The model under review builds one solid part; all positions refer to its coordinate system, in mm. A direction names the side the tool comes from. Round coordinates to 2 decimals unless told otherwise and drop trailing zeros. Order: outer loops, then holes, each group sorted by start corner. A loop starts at its lowest first (then second) coordinate and runs counter-clockwise, first axis right, second up.
Autodesk Inventor part; units mm, degrees
ref_plane "YZ Plane" through (0, 0, 0) normal (1, 0, 0) x (0, 1, 0)
ref_plane "XZ Plane" through (0, 0, 0) normal (0, 1, 0) x (-1, 0, 0)
ref_plane "XY Plane" through (0, 0, 0) normal (0, 0, 1) x (1, 0, 0)
sketch "Sketch1" plane through (0, 0, 0) normal (0, 0, 1) x (1, 0, 0)
  circle A0 centre (0, 0) radius 100
  dimension "Dia" = 200
extrude "Extrusion1" add sketch "Sketch1" along normal blind 25
sketch "Sketch2" plane through (0, 0, 25) normal (0, 0, 1) x (1, 0, 0)
  line L0 (-100, 12.5) -> (100, 12.5)
  line L1 (100, 12.5) -> (100, -12.5)
  line L2 (100, -12.5) -> (-100, -12.5)
  line L3 (-100, -12.5) -> (-100, 12.5)
  line L4 (-100, 12.5) -> (100, -12.5) construction
  line L5 (100, 12.5) -> (-100, -12.5) construction
  point P0 (0, 0)
  dimension "d3" = 200
  dimension "d4" = 25
extrude "Extrusion2" cut sketch "Sketch2" against normal blind 10 draft 12
pattern_circular "Circular Pattern1" count 2 over 90 about axis through (0, 0, 0) along (0, 0, 1) of "Extrusion2"
equation "\"d3\" = Dia"
(1) Consider section B-B (z = 19.25). Write out the cut boundary in (x, y), and give its area (3 significant figures).
Data:
outline: (-99.05, -13.72) arc R100 ccw to (-13.72, -99.05) - (-13.72, -13.72) - close; (-99.05, 13.72) - (-13.72, 13.72) - (-13.72, 99.05) arc R100 ccw to start; (13.72, -99.05) arc R100 ccw to (99.05, -13.72) - (13.72, -13.72) - close; (13.72, 13.72) - (99.05, 13.72) arc R100 ccw to (13.72, 99.05) - close
area: 21,200 mm2
(2) Insertion check: pin 1 (8 mm diameter, centred on x = 33, z = 14, fed in from +Y); pin 2 (4 mm diameter, centred on y = 34, z = 11.5, fed in from +X); pin 3 (6 mm diameter, centred on x = 13.5, z = 4, fed in from +Y); pin 4 (2 mm diameter, centred on x = -61, y = 43.5, fed in from -Z). Each pin has a flat end and moves straight along its axis. Give the tip position at first contact, or say it passes through.
Data:
pin 1: stops at y = 95.7
pin 2: stops at x = 94.74
pin 3: stops at y = 99.45
pin 4: stops at z = 0
(3) For faces 1 (the flat face through (0, -7, 15)), 2 (the flat face through (46, 47, 25)), list the 3-axis set-ups (+Z, -Z, +X, -X, +Y, -Y) from which the entire face can be reached by the end or side of a thin tool; tool diameter is ignored.
Data:
face 1: none
face 2: +Z, +X, -X, +Y, -Y
(4) Draft analysis for pull direction X (two halves, no side actions). For faces 3 (the flat face through (13.548, -55.251, 20.07)), 4 (the flat face through (-1, 1, 0)), 5 (the cylindrical face through (92.375, 38.301, 12.325)), state which applies: pulls with the +X half, pulls with the -X half, needs draft (parallel to the pull), parting line crosses it, or undercut.
Data:
face 3: undercut
face 4: needs draft
face 5: parting line crosses it
(5) To check wall thickness, follow probe 1 along Z at (x, y) = (-0.5, 44.5); probe 2 along Y at (x, z) = (67, 17.75); probe 3 along Y at (x, z) = (-82, 20.5). State the ranges of each line that lie inside material, in increasing order.
Data:
probe 1: z = 0 to 15
probe 2: y = -74.24 to -14.04, 14.04 to 74.24
probe 3: y = -57.24 to -13.46, 13.46 to 57.24
(6) Consider section C-C (x = -21). Write out the cut boundary in (y, z).
Data:
outline: (-97.77, 0) - (97.77, 0) - (97.77, 25) - (12.5, 25) - (14.63, 15) - (-14.63, 15) - (-12.5, 25) - (-97.77, 25) - close
(7) Consider section D-D (z = 8.75). Write out the cut boundary in (x, y).
Data:
outline: circle Ø200 at (0, 0)
(8) Consider section A-A (y = -60). Write out the cut boundary in (x, z).
Data:
outline: (-80, 0) - (80, 0) - (80, 25) - (12.5, 25) - (14.63, 15) - (-14.63, 15) - (-12.5, 25) - (-80, 25) - close
